from build123d import *

# Parameters (mm, degrees)
SCHIZZO1_R                                           = 21.5
ESTRUSIONE_ESTRUSIONE1_DEPTH                         = 20
FORO_LAMATO_PER_VITE_M6_A_TESTA_CILINDRI_D           = 6.6
FORO_LAMATO_PER_VITE_M6_A_TESTA_CILINDRI_CBORE_D     = 11
FORO_LAMATO_PER_VITE_M6_A_TESTA_CILINDRI_CBORE_DEPTH = 6.4
FORO_LAMATO_PER_VITE_M6_A_TESTA_CILI_2_D             = 6.6
FORO_LAMATO_PER_VITE_M6_A_TESTA_CILI_2_CBORE_D       = 11
FORO_LAMATO_PER_VITE_M6_A_TESTA_CILI_2_CBORE_DEPTH   = 6.4
SCHIZZO7_W                                           = 15.52137419
SCHIZZO7_H                                           = 2
TAGLIO_ESTRUSIONE1_DEPTH                             = 140.373598648


with BuildPart() as part:
    # Schizzo1 → Estrusione-Estrusione1 (new body)
    with BuildSketch(Plane.XY):
        Polygon((0, 0), (100, 0), (100, 20), (81, 20), (81, 95), (19, 95), (19, 20), (0, 20), align=None)
        with Locations((50, 65)):
            Circle(SCHIZZO1_R, mode=Mode.SUBTRACT)
    extrude(amount=ESTRUSIONE_ESTRUSIONE1_DEPTH)

    # Foro lamato per Vite M6 a testa cilindri (through all)
    with Locations(Plane(origin=(9.5, 20, 10), x_dir=(0, 0, 1), z_dir=(0, 1, 0))):
        with Locations((0, 0), (0, 81)):
            CounterBoreHole(FORO_LAMATO_PER_VITE_M6_A_TESTA_CILINDRI_D / 2, FORO_LAMATO_PER_VITE_M6_A_TESTA_CILINDRI_CBORE_D / 2, FORO_LAMATO_PER_VITE_M6_A_TESTA_CILINDRI_CBORE_DEPTH)

    # Foro lamato per Vite M6 a testa cili 2 (through all)
    with Locations(Plane(origin=(25, 95, 10), x_dir=(0, 0, 1), z_dir=(0, 1, 0))):
        with Locations((0, 0)):
            CounterBoreHole(FORO_LAMATO_PER_VITE_M6_A_TESTA_CILI_2_D / 2, FORO_LAMATO_PER_VITE_M6_A_TESTA_CILI_2_CBORE_D / 2, FORO_LAMATO_PER_VITE_M6_A_TESTA_CILI_2_CBORE_DEPTH)

    # Schizzo7 → Taglio-Estrusione1 (cut, through all)
    with BuildSketch(Plane(origin=(0, 0, 0), x_dir=(-1, 0, 0), z_dir=(0, 0, -1))):
        with Locations((-23.66540179, 65)):
            Rectangle(SCHIZZO7_W, SCHIZZO7_H)
    extrude(amount=-TAGLIO_ESTRUSIONE1_DEPTH, mode=Mode.SUBTRACT)


solid = part.part
Could you check a few things on this model? Use its own coordinates, in mm. A direction names the side the tool comes from. Give positions to 0.01 mm unless a question says otherwise; leave off trailing zeros. Write each loop counter-clockwise with the first axis right and the second up, starting at its lowest first coordinate (ties: lowest second). Pieces come first, ordered by that corner, then holes. Notation, with made-up numbers: (68, -36) -> (111, -36) arc R33 cw to (111, -1) -> close; hole circle Ø9 at (40, 43). An arc over 180 degrees is marked (long way). Answer as a JSON object with one key per item and string values.
Q1. Suppose I cut it at A-A on y = 45. Write out the boundary of the cut face in (x, z), then the cut area to 3 significant figures.
Taken from the geometry:
{"outline": "(19, 0) -> (42.11, 0) -> (42.11, 20) -> (19, 20) -> close; (57.89, 0) -> (81, 0) -> (81, 20) -> (57.89, 20) -> close; hole circle Ø6.6 at (25, 10)", "area": "890 mm²"}
Q2. Which directions (+Z, -Z, +X, -X, +Y, -Y) give clear straight access to the entire face, cutting with the end or side of a thin tool? Please do faces 1 (the flat face through (14, 20, 5)), 2 (the flat face through (86, 20, 5)), 3 (the flat face through (22, 66, 8)), 4 (the flat face through (49, 38, 20)), 5 (the flat face through (10, 13.6, 14)).
Taken from the geometry:
{"face 1": "+Z, -Z, -X, +Y", "face 2": "+Z, -Z, +X, +Y", "face 3": "+Z, -Z, -X", "face 4": "+Z, +X, -X, +Y, -Y", "face 5": "+Y"}
Q3. Will these pins go through, and if not, where does the flat tip stop? pin 1 Ø3 at (y, z) = (14, 2.5) entering from -X; pin 2 Ø8 at (x, z) = (88, 7) entering from +Y; pin 3 Ø3 at (x, z) = (23.5, 11.5) entering from +Y; pin 4 Ø5 at (y, z) = (52, 14) entering from -X.
Taken from the geometry:
{"pin 1": "stops at x = 0", "pin 2": "stops at y = 20", "pin 3": "stops at y = 88.6", "pin 4": "stops at x = 19"}
Q4. Suppose I cut it at B-B on x = 90.5. Write out the boundary of the cut face in (y, z), then the cut area to 3 significant figures.
Taken from the geometry:
{"outline": "(0, 0) -> (20, 0) -> (20, 4.5) -> (13.6, 4.5) -> (13.6, 6.7) -> (0, 6.7) -> close; (0, 13.3) -> (13.6, 13.3) -> (13.6, 15.5) -> (20, 15.5) -> (20, 20) -> (0, 20) -> close", "area": "240 mm²"}
Q5. Suppose I cut it at C-C on y = 8.5. Write out the boundary of the cut face in (x, z), then the cut area to 3 significant figures.
Taken from the geometry:
{"outline": "(0, 0) -> (100, 0) -> (100, 20) -> (0, 20) -> close; hole circle Ø6.6 at (9.5, 10); hole circle Ø6.6 at (25, 10); hole circle Ø6.6 at (90.5, 10)", "area": "1,900 mm²"}
Q6. Please list where these lines run through material, in increasing order: L1, parallel to X at y = 7.25, z = 10; L2, parallel to X at y = 15.5, z = 10; L3, parallel to X at y = 24, z = 10.
Taken from the geometry:
{"L1": "x = 0 to 6.2, 12.8 to 21.7, 28.3 to 87.2, 93.8 to 100", "L2": "x = 0 to 4, 15 to 21.7, 28.3 to 85, 96 to 100", "L3": "x = 19 to 21.7, 28.3 to 81"}
Q7. We'd pull the mould along X, two halves only. Please class faces 6 (the flat face through (49, 38, 0)), 7 (the cylindrical face through (7.39, 16.84, 15.08)), 8 (the flat face through (100, 10, 10)): released by +X, released by -X, zero draft, split by the parting line, or undercut.
Taken from the geometry:
{"face 6": "zero draft", "face 7": "undercut", "face 8": "released by +X"}
Q8. Suppose I cut it at D-D on x = 25. Write out the boundary of the cut face in (y, z).
Taken from the geometry:
{"outline": "(0, 0) -> (64, 0) -> (64, 6.7) -> (0, 6.7) -> close; (0, 13.3) -> (64, 13.3) -> (64, 20) -> (0, 20) -> close; (66, 0) -> (95, 0) -> (95, 4.5) -> (88.6, 4.5) -> (88.6, 6.7) -> (66, 6.7) -> close; (66, 13.3) -> (88.6, 13.3) -> (88.6, 15.5) -> (95, 15.5) -> (95, 20) -> (66, 20) -> close"}
